```python
from build123d import *

# Parameters (mm, degrees)
SKETCH1_W           = 190
SKETCH1_H           = 225
SKETCH1_W_2         = 90
SKETCH1_H_2         = 125
SKETCH1_W_3         = 45
SKETCH1_H_3         = 13.183655632
BOSS_EXTRUDE1_DEPTH = 3
SKETCH1_3_W         = 190
SKETCH1_3_H         = 225
SKETCH1_3_W_2       = 90
SKETCH1_3_H_2       = 125
SKETCH1_3_W_3       = 45
SKETCH1_3_H_3       = 13.183655632
BOSS_EXTRUDE2_DEPTH = 10


with BuildPart() as part:
    # Sketch1 → Boss-Extrude1 (new body)
    # profile 1 of 3: a face of its own
    with BuildSketch(Plane(origin=(0, 0, 0), x_dir=(1, 0, 0), z_dir=(0, 1, 0))):
        with Locations((85, 102.5)):
            Rectangle(SKETCH1_W, SKETCH1_H)
        with Locations((45, 62.5)):
            Rectangle(SKETCH1_W_2, SKETCH1_H_2, mode=Mode.SUBTRACT)
    # profile 2 of 3: a face of its own
    with BuildSketch(Plane(origin=(0, 0, 0), x_dir=(1, 0, 0), z_dir=(0, 1, 0))):
        with Locations((45, 62.5)):
            Rectangle(SKETCH1_W_2, SKETCH1_H_2)
    # profile 3 of 3: a face of its own
    with BuildSketch(Plane(origin=(0, 0, 0), x_dir=(1, 0, 0), z_dir=(0, 1, 0))):
        with Locations((45, -16.591827816)):
            Rectangle(SKETCH1_W_3, SKETCH1_H_3)
    extrude(amount=-BOSS_EXTRUDE1_DEPTH)

    # Sketch1_3 → Boss-Extrude2 (add)
    # profile 1 of 2: a face of its own
    with BuildSketch(Plane(origin=(0, 0, 0), x_dir=(1, 0, 0), z_dir=(0, 1, 0))):
        with Locations((85, 102.5)):
            Rectangle(SKETCH1_3_W, SKETCH1_3_H)
        with Locations((45, 62.5)):
            Rectangle(SKETCH1_3_W_2, SKETCH1_3_H_2, mode=Mode.SUBTRACT)
    # profile 2 of 2: a face of its own
    with BuildSketch(Plane(origin=(0, 0, 0), x_dir=(1, 0, 0), z_dir=(0, 1, 0))):
        with Locations((45, -16.591827816)):
            Rectangle(SKETCH1_3_W_3, SKETCH1_3_H_3)
    extrude(amount=BOSS_EXTRUDE2_DEPTH)


solid = part.part
```
Verification items for the finished model (mm, model axes). A direction names the side the tool comes from. Coordinates: 2 decimals unless noted, no trailing zeros. Order: outer loops, then holes, each group sorted by start corner. A loop starts at its lowest first (then second) coordinate and runs counter-clockwise, first axis right, second up. Notation, with made-up numbers: (49.5, 75) - (107.5, 75) arc R14 ccw to (107.5, 83) - close; hole circle Ø6 at (-18.75, 19.25). An arc over 180 degrees is marked (long way). Return JSON: item names as keys, results as strings.
(1) Section check C-C, the plane x = 55. Record the cut outline in (y, z), and give its area (3 significant figures).
Filled sheet:
{"outline": "(-3, -215) - (10, -215) - (10, -125) - (0, -125) - (0, 0) - (10, 0) - (10, 23.18) - (-3, 23.18) - close", "area": "1,850 mm^2"}
(2) Mould release check, pull along Z, two halves, no side actions. Record for faces 6 (the flat face through (44, 5, -125)), 7 (the flat face through (105, 10, -98)), 8 (the flat face through (123, 3, 10)): pulls with the +Z half, pulls with the -Z half, needs draft (parallel to the pull), parting line crosses it, or undercut.
Filled sheet:
{"face 6": "undercut", "face 7": "needs draft", "face 8": "pulls with the +Z half"}
(3) Section check D-D, the plane x = 116. Record the cut outline in (y, z).
Filled sheet:
{"outline": "(-3, -215) - (10, -215) - (10, 10) - (-3, 10) - close"}
(4) Section check B-B, the plane z = -8.5. Record the cut outline in (x, y), and give its area (3 significant figures).
Filled sheet:
{"outline": "(-10, -3) - (180, -3) - (180, 10) - (90, 10) - (90, 0) - (0, 0) - (0, 10) - (-10, 10) - close", "area": "1,570 mm^2"}
(5) Section check A-A, the plane y = 3. Record the cut outline in (x, z), and give its area (3 significant figures).
Filled sheet:
{"outline": "(-10, -215) - (180, -215) - (180, 10) - (67.5, 10) - (67.5, 23.18) - (22.5, 23.18) - (22.5, 10) - (-10, 10) - close; hole (0, -125) - (90, -125) - (90, 0) - (0, 0) - close", "area": "32,100 mm^2"}
(6) Thickness scan on line 1 along Z through (x, y) = (83.5, 7.5); line 2 along Z through (x, y) = (44.5, 2.75); line 3 along X through (y, z) = (2, -118). Record the ranges inside material, lowest first.
Filled sheet:
{"line 1": "z = -215 to -125, 0 to 10", "line 2": "z = -215 to -125, 0 to 23.18", "line 3": "x = -10 to 0, 90 to 180"}
(7) Access from +Z, -Z, +X, -X, +Y, -Y to the whole of each face (thin tool, end or side, straight path). Record for faces 1 (the flat face through (84, -3, -98)), 2 (the flat face through (44, 5, 0)), 3 (the flat face through (67.5, 4, 17)), 4 (the flat face through (22.5, 3, 17)), 5 (the flat face through (180, 3, -101)).
Filled sheet:
{"face 1": "+Z, -Z, +X, -X, -Y", "face 2": "+Y", "face 3": "+Z, +X, +Y, -Y", "face 4": "+Z, -X, +Y, -Y", "face 5": "+Z, -Z, +X, +Y, -Y"}
(8) Go/stop test with flat-tipped pins: pin 1 (4 mm diameter, centred on x = 8, y = 5, fed in from +Z); pin 2 (6.5 mm diameter, centred on y = 6.5, z = 18, fed in from -X). Record where each tip stops, or that it passes through.
Filled sheet:
{"pin 1": "stops at z = 10", "pin 2": "stops at x = 22.5"}
